Check sheet for the modelled part. Datum: model origin and axes. Units: mm. Give positions to 0.01 mm unless a question says otherwise; leave off trailing zeros. Write each loop counter-clockwise with the first axis right and the second up, starting at its lowest first coordinate (ties: lowest second). Pieces come first, ordered by that corner, then holes. Notation, with made-up numbers: M 5,12 L 31,12 A18 ccw 31,33 Z; hole C 14,51.25 d5. An arc over 180 degrees is marked long. Write each question's results on one line, items separated by ' | '. Start each with the question number.
Autodesk Inventor part; units mm, degrees
ref_plane "YZ Plane" through (0, 0, 0) normal (1, 0, 0) x (0, 1, 0)
ref_plane "XZ Plane" through (0, 0, 0) normal (0, 1, 0) x (-1, 0, 0)
ref_plane "XY Plane" through (0, 0, 0) normal (0, 0, 1) x (1, 0, 0)
sketch "Base" plane through (0, 0, 0) normal (0, 1, 0) x (-1, 0, 0)
  line L0 (0, 0) -> (-117, 0)
  line L1 (-117, 0) -> (-117, -85)
  line L2 (-117, -85) -> (0, -85)
  line L3 (0, -85) -> (0, 0)
  line L4 (-117, -85) -> (-112, -85)
  line L5 (-112, -85) -> (-112, 0)
  line L6 (-112, 0) -> (-117, 0)
  line L7 (-117, 0) -> (-117, -85)
  line L8 (-112, -85) -> (-57, -85)
  line L9 (-57, -85) -> (-57, 0)
  line L10 (-57, 0) -> (-112, 0)
  line L11 (-112, 0) -> (-112, -85)
  line L12 (-57, -75) -> (-27, -75)
  line L13 (-27, -75) -> (-27, -10)
  line L14 (-27, -10) -> (-57, -10)
  line L15 (-57, -10) -> (-57, -75)
  circle A0 centre (-30.5, -71.5) radius 1.3
  circle A1 centre (-53.5, -71.5) radius 1.3
  circle A2 centre (-30.5, -13.5) radius 1.3
  circle A3 centre (-53.5, -13.5) radius 1.3
  line L16 (-27, -85) -> (-27, 0)
  line L17 (0, -83.35) -> (-50, -83.35)
  line L18 (-50, -83.35) -> (-50, -1.65)
  line L19 (-50, -1.65) -> (0, -1.65)
  line L20 (0, -1.65) -> (0, -83.35)
  circle A4 centre (-2.9, -80.45) radius 1.55
  circle A5 centre (-47.1, -80.45) radius 1.55
  circle A6 centre (-47.1, -4.55) radius 1.55
  circle A7 centre (-2.9, -4.55) radius 1.55
  line L21 (-50, -17.1) -> (-57, -17.1)
  line L22 (-57, -17.1) -> (-57, -67.9)
  line L23 (-57, -67.9) -> (-50, -67.9)
  line L24 (-50, -67.9) -> (-50, -17.1)
  line L25 (-50, -17.1) -> (-57, -67.9) construction
  line L26 (-57, -17.1) -> (-50, -67.9) construction
  line L27 (-7.22, -1.65) -> (-42.78, -1.65)
  line L28 (-42.78, -1.65) -> (-42.78, -5.15)
  line L29 (-42.78, -5.15) -> (-7.22, -5.15)
  line L30 (-7.22, -5.15) -> (-7.22, -1.65)
  point P0 (-27, -10)
  point P1 (-53.5, -42.5)
  dimension "d0" = 117
  dimension "d1" = 85
  dimension "d2" = 5
  dimension "d3" = 85
  dimension "d10" = 55
  dimension "d11" = 85
  dimension "d12" = 30
  dimension "d13" = 65
  dimension "d14" = 10
  dimension "d15" = 10
  dimension "d16" = 2.6
  dimension "d17" = 2.6
  dimension "d18" = 2.6
  dimension "d19" = 2.6
  dimension "d20" = 3.5
  dimension "d21" = 3.5
  dimension "d22" = 3.5
  dimension "d23" = 3.5
  dimension "d24" = 3.5
  dimension "d25" = 3.5
  dimension "d26" = 3.5
  dimension "d27" = 3.5
  dimension "d28" = 0
  dimension "d38" = 50
  dimension "d39" = 81.7
  dimension "d40" = 1.65
  dimension "d41" = 1.65
  dimension "d42" = 3.1
  dimension "d43" = 3.1
  dimension "d44" = 3.1
  dimension "d45" = 3.1
  dimension "d46" = 2.9
  dimension "d48" = 2.9
  dimension "d49" = 2.9
  dimension "d50" = 2.9
  dimension "d51" = 2.9
  dimension "d52" = 2.9
  dimension "d53" = 2.9
  dimension "d54" = 50.8
  dimension "d55" = 7
  dimension "d56" = 29
  dimension "d57" = 29
  dimension "d63" = 2.9
  dimension "d64" = 35.56
  dimension "d65" = 3.5
  dimension "d66" = 7.22
  dimension "d67" = 7.22
  dimension "d71" = 44.2
  dimension "d72" = 75.9
extrude "Extrusion4" add sketch "Base" along normal blind 3 contours L14 L18 L21 L9 | L14 L13 L12 L18 | L23 L18 L12 L9
fillet "Fillet6" radius 2 6 edges at (27, 1.5, -10) (57, 1.5, -10) (57, 1.5, -17.1) (57, 1.5, -67.9) (57, 1.5, -75) (27, 1.5, -75)
properties part number "00_BottomPart"
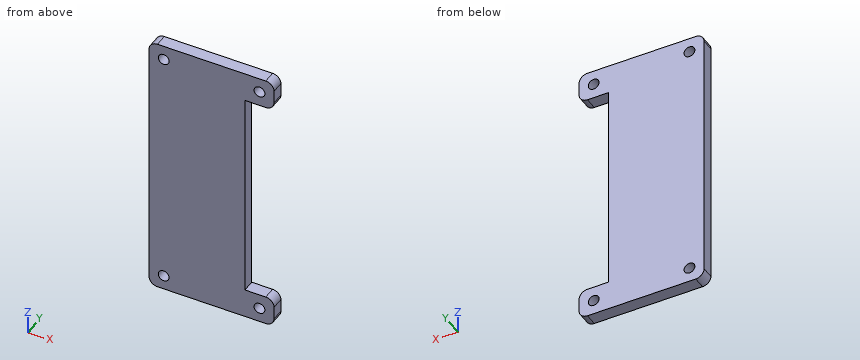
Q1. Section check C-C on x = 30.5. Record the boundary of the cut face in (y, z), plus the area to 3 significant figures.
Q2. Scan lines: L1, parallel to Z at x = 30.5, y = 0.95; L2, parallel to X at y = 2.25, z = -71.5; L3, parallel to Z at x = 53.5, y = 1. Record each from-to range of solid material in increasing order.
Q3. Section check D-D on y = 0.6. Record the boundary of the cut face in (x, z).
Q4. Section check B-B on z = -13.5. Record the boundary of the cut face in (x, y), plus the area to 3 significant figures.
Q5. Depth check by flat-ended pin: pin 1 Ø1.6 at (x, z) = (53.5, -13.5) entering from -Y. Enter the tip coordinate at first touch or a pass-through.
Q6. Section check A-A on x = 53.5. Record the boundary of the cut face in (y, z).
Check result:
1) outline: M 0,-75 L 3,-75 L 3,-72.8 L 0,-72.8 Z; M 0,-70.2 L 3,-70.2 L 3,-14.8 L 0,-14.8 Z; M 0,-12.2 L 3,-12.2 L 3,-10 L 0,-10 Z | area: 179 mm^2
2) L1: -75 to -72.8, -70.2 to -14.8, -12.2 to -10 | L2: 27 to 29.2, 31.8 to 52.2, 54.8 to 57 | L3: -75 to -72.8, -70.2 to -67.9, -17.1 to -14.8, -12.2 to -10
3) outline: M 27,-73 A2 ccw 29,-75 L 55,-75 A2 ccw 57,-73 L 57,-69.9 A2 ccw 55,-67.9 L 50,-67.9 L 50,-17.1 L 55,-17.1 A2 ccw 57,-15.1 L 57,-12 A2 ccw 55,-10 L 29,-10 A2 ccw 27,-12 Z; hole C 30.5,-71.5 d2.6; hole C 30.5,-13.5 d2.6; hole C 53.5,-71.5 d2.6; hole C 53.5,-13.5 d2.6
4) outline: M 27,0 L 29.2,0 L 29.2,3 L 27,3 Z; M 31.8,0 L 52.2,0 L 52.2,3 L 31.8,3 Z; M 54.8,0 L 57,0 L 57,3 L 54.8,3 Z | area: 74.4 mm^2
5) pin 1: through
6) outline: M 0,-75 L 3,-75 L 3,-72.8 L 0,-72.8 Z; M 0,-70.2 L 3,-70.2 L 3,-67.9 L 0,-67.9 Z; M 0,-17.1 L 3,-17.1 L 3,-14.8 L 0,-14.8 Z; M 0,-12.2 L 3,-12.2 L 3,-10 L 0,-10 Z
